For this review, take the finished solid that the model builds, in its own axes (mm). Face numbers are marked on the shaded views. A direction names the side the tool comes from. Round coordinates to 2 decimals unless told otherwise and drop trailing zeros. Loops run counter-clockwise (first coordinate to the right, second up) from the corner with the lowest first, then second, coordinate; pieces in that order, holes last. Notation, with made-up numbers: (76.5, 80.5) -> (121.5, 80.5) arc R30 cw to (121.5, 110.5) -> close; hole circle Ø1 at (45.25, 43.25). An arc over 180 degrees is marked (long way). Write each question's results on one line, items separated by ' | '.
```python
from build123d import *

# Parameters (mm, degrees)
SKETCH_1_R          = 2.85
EXTRUDE_1_DEPTH     = 3
SKETCH_2_R          = 1.5
EXTRUDE_2_DEPTH     = 12
SKETCH_3_R          = 1.29
CUT_EXTRUDE_1_DEPTH = 1.3
FILLET_1_R          = 0.3
CHAMFER_1_SIZE      = 0.3
CHAMFER_2_SIZE      = 0.15


with BuildPart() as part:
    # 草图1 → 凸台-拉伸1 (new body)
    with BuildSketch(Plane(origin=(0, 0, 0), x_dir=(1, 0, 0), z_dir=(0, 1, 0))):
        with Locations(Location((0, 0, 0), (0, 0, 270))):
            Circle(SKETCH_1_R)
    extrude(amount=EXTRUDE_1_DEPTH)

    # 草图2 → 凸台-拉伸2 (add)
    with BuildSketch(Plane(origin=(0, 3, 0), x_dir=(1, 0, 0), z_dir=(0, 1, 0))):
        with Locations(Location((0, 0, 0), (0, 0, 270))):
            Circle(SKETCH_2_R)
    extrude(amount=EXTRUDE_2_DEPTH)

    # 草图3 → 切除-拉伸1 (cut)
    with BuildSketch(Plane.XZ):
        with Locations(Location((0, 0, 0), (0, 0, 270))):
            Circle(SKETCH_3_R)
    extrude(amount=-CUT_EXTRUDE_1_DEPTH, mode=Mode.SUBTRACT)

    # 圆角1
    fillet_1_edges = [part.edges().sort_by_distance(p)[0] for p in [
        (0, 0, -2.85),
        (0, 3, -2.85),
    ]]
    fillet(fillet_1_edges, radius=FILLET_1_R)

    # 倒角1
    chamfer_1_edges = [part.edges().sort_by_distance(p)[0] for p in [
        (0, 15, -1.5),
    ]]
    chamfer(chamfer_1_edges, length=CHAMFER_1_SIZE)

    # 倒角2
    chamfer_2_edges = [part.edges().sort_by_distance(p)[0] for p in [
        (0, 0, 1.29),
    ]]
    chamfer(chamfer_2_edges, length=CHAMFER_2_SIZE)


solid = part.part
```
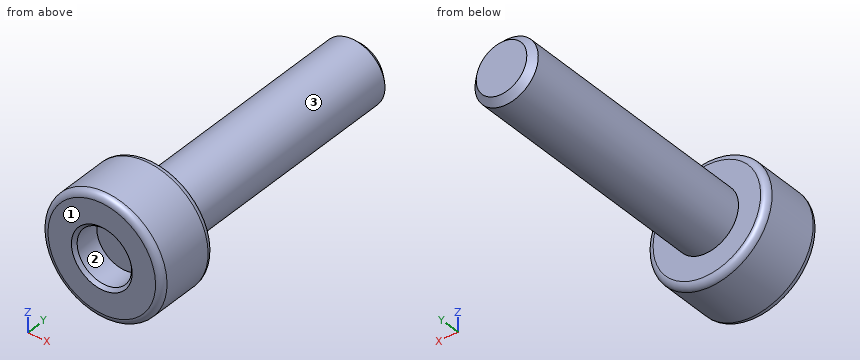
1. Consider section B-B (z = 0). State the section outline as (x, y) points.
Values found:
outline: (-2.85, 0.3) arc R0.3 ccw to (-2.55, 0) -> (-1.44, 0) -> (-1.29, 0.15) -> (-1.29, 1.3) -> (1.29, 1.3) -> (1.29, 0.15) -> (1.44, 0) -> (2.55, 0) arc R0.3 ccw to (2.85, 0.3) -> (2.85, 2.7) arc R0.3 ccw to (2.55, 3) -> (1.5, 3) -> (1.5, 14.7) -> (1.2, 15) -> (-1.2, 15) -> (-1.5, 14.7) -> (-1.5, 3) -> (-2.55, 3) arc R0.3 ccw to (-2.85, 2.7) -> close
2. Consider section A-A (x = 0). State the section outline as (y, z) points, plus the area to 3 significant figures.
Values found:
outline: (0, -2.55) arc R0.3 ccw to (0.3, -2.85) -> (2.7, -2.85) arc R0.3 ccw to (3, -2.55) -> (3, -1.5) -> (14.7, -1.5) -> (15, -1.2) -> (15, 1.2) -> (14.7, 1.5) -> (3, 1.5) -> (3, 2.55) arc R0.3 ccw to (2.7, 2.85) -> (0.3, 2.85) arc R0.3 ccw to (0, 2.55) -> (0, 1.44) -> (0.15, 1.29) -> (1.3, 1.29) -> (1.3, -1.29) -> (0.15, -1.29) -> (0, -1.44) -> close | area: 49.6 mm2
3. Tool access review of the marked faces 1, 2 and 3: name each direction out of +Z, -Z, +X, -X, +Y, -Y from which nothing blocks a thin tool from reaching the whole face with its end or side.
Values found:
face 1: +Z, -Z, +X, -X, -Y | face 2: -Y | face 3: +Y
4. Consider section C-C (y = 12.5). State the section outline as (x, z) points.
Values found:
outline: circle Ø3 at (0, 0)
5. To check wall thickness, follow probe 1 along X at (y, z) = (1.1, 0); probe 2 along Y at (x, z) = (-1.1, -0.25); probe 3 along Y at (x, z) = (2.05, -0.4). State the ranges of each line that lie inside material, in increasing order.
Values found:
probe 1: x = -2.85 to -1.29, 1.29 to 2.85 | probe 2: y = 1.3 to 15 | probe 3: y = 0 to 3
6. For pin 1 (3 mm diameter, centred on x = 0, z = 0.5, fed in from -Y); pin 2 (2 mm diameter, centred on x = 1, y = 8, fed in from -Z); pin 3 (3 mm diameter, centred on y = 7, z = 1, fed in from -X); pin 4 (1.5 mm diameter, centred on y = 11.5, z = 0.5, fed in from +X), all flat-tipped, find the tip position at first contact; note any pin that passes through.
Values found:
pin 1: stops at y = 0 | pin 2: stops at z = -1.5 | pin 3: stops at x = -1.5 | pin 4: stops at x = 1.5
